Drawing for the job (mm, zero at the part's lowest x, y, z). A direction names the side the tool comes from. Give positions to 0.01 mm unless a question says otherwise; leave off trailing zeros. Loops run counter-clockwise (first coordinate to the right, second up) from the corner with the lowest first, then second, coordinate; pieces in that order, holes last.
1) Band-saw the part on C-C on x = 69. List the corners of the cut face in (y, z).
2) Two-plate mould, pull along X, no slides. Class the marked faces 1, 2 and 3: +X half, -X half, draft (parallel to the pull), parting line (faces both ways), or undercut.
3) Band-saw the part on A-A on x = 40. List the corners of the cut face in (y, z).
4) 3-axis set-ups, long thin cutter, end or side, ignore diameter. For the marked faces 4, 5 and 6: which of +Z, -Z, +X, -X, +Y, -Y reach the whole face in a straight line?
5) Flat gauge pins, fed straight in: P1, Ø2, axis at x = 15.5, z = 4, coming from the +Y side; P2, Ø3, axis at y = 96, z = 2.5, coming from the -X side. Where does each tip first touch, or does it go through?
6) Band-saw the part on B-B on z = 2.75. List the corners of the cut face in (x, y).
7) Wall check: line 1 (X direction, y = 110, z = 7.5); line 2 (Y direction, x = 40, z = 4.75); line 3 (Y direction, x = 47, z = 8) (3 decimals). Give the ranges that are in metal, low to high.
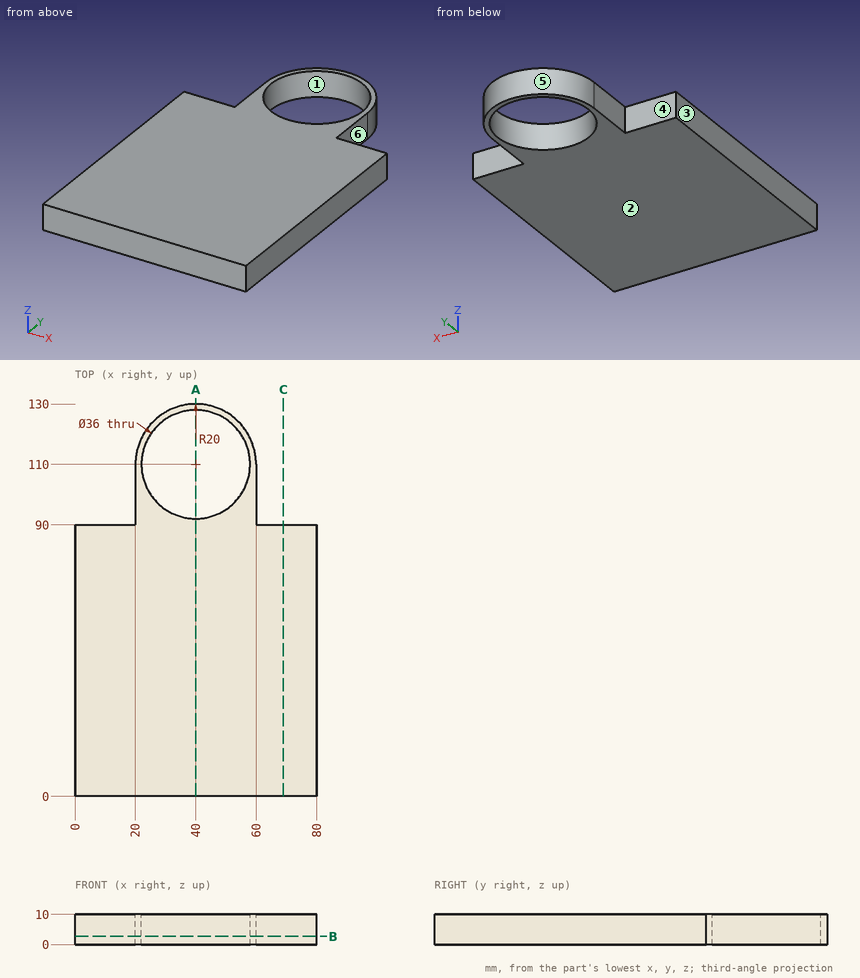
Findings below:
1. outline: (0, 0) - (90, 0) - (90, 10) - (0, 10) - close
2. face 1: undercut
2. face 2: draft
2. face 3: -X half
3. outline: (0, 0) - (92, 0) - (92, 10) - (0, 10) - close; (128, 0) - (130, 0) - (130, 10) - (128, 10) - close
4. face 4: +Z, -Z, -X, +Y
4. face 5: +Z, -Z, +Y
4. face 6: +Z, -Z, +X, +Y
5. P1: stops at y = 90
5. P2: stops at x = 20
6. outline: (0, 0) - (80, 0) - (80, 90) - (60, 90) - (60, 110) arc R20 ccw to (20, 110) - (20, 90) - (0, 90) - close; hole circle Ø36 at (40, 110)
7. line 1: x = 20 to 22, 58 to 60
7. line 2: y = 0 to 92, 128 to 130
7. line 3: y = 0 to 93.417, 126.583 to 128.735
